from build123d import *

# Parameters (mm, degrees)
SKETCH_W                   = 21.1
SKETCH_H                   = 43.6
PAD_DEPTH                  = 3
SKETCH004_W                = 23.1
SKETCH004_H                = 45.6
PAD001_DEPTH               = 3
SKETCH005_W                = 7.05
SKETCH005_H                = 1.1
PAD002_DEPTH               = 5
SKETCH005_MIRRORED002_2_W  = 7.05
SKETCH005_MIRRORED002_2_H  = 1.1
PAD002_MIRRORED002_2_DEPTH = 5
SKETCH002_W                = 4.6
SKETCH002_H                = 9.5
POCKET_DEPTH               = 1
SKETCH001_R                = 1.65
POCKET001_DEPTH            = 0.001
POCKET001_DEPTH_BACK       = -5.001
SKETCH003_W                = 4
SKETCH003_H                = 4
POCKET002_DEPTH            = 2
SKETCH003_MIRRORED_2_W     = 4
SKETCH003_MIRRORED_2_H     = 4
POCKET002_MIRRORED_2_DEPTH = 2


with BuildPart() as part:
    # Sketch → Pad (new body)
    with BuildSketch(Plane.XY):
        Rectangle(SKETCH_W, SKETCH_H)
    extrude(amount=PAD_DEPTH)

    # Sketch004 → Pad001 (join)
    with BuildSketch(Plane.XY):
        Rectangle(SKETCH004_W, SKETCH004_H)
    extrude(amount=PAD001_DEPTH)

    # Sketch005 → Pad002 (join)
    with BuildSketch(Plane.XY):
        with Locations((3.525, 23.35)):
            Rectangle(SKETCH005_W, SKETCH005_H)
        Polygon((11.55, 22.8), (10.55, 22.8), (10.55, 23.9), (12.65, 23.9), (12.65, 0), (11.55, 0), align=None)
    pad002 = extrude(amount=PAD002_DEPTH)

    # Sketch005 Mirrored002 2 → Pad002 Mirrored002 2 (add)
    with BuildSketch(Plane(origin=(0, 0, 0), x_dir=(-1, 0, 0), z_dir=(0, 0, -1))):
        with Locations((3.525, 23.35)):
            Rectangle(SKETCH005_MIRRORED002_2_W, SKETCH005_MIRRORED002_2_H)
        Polygon((11.55, 22.8), (10.55, 22.8), (10.55, 23.9), (12.65, 23.9), (12.65, 0), (11.55, 0), align=None)
    pad002_mirrored002_2 = extrude(amount=-PAD002_MIRRORED002_2_DEPTH)

    # Mirrored003: Pad002, Pad002 Mirrored002 2 across Sketch005 H_Axis
    add(pad002.mirror(Plane.ZX))
    add(pad002_mirrored002_2.mirror(Plane.ZX))

    # Sketch002 → Pocket (cut)
    with BuildSketch(Plane(origin=(-8.2, 8.2, 3), x_dir=(1, 0, 0), z_dir=(0, 0, 1))):
        Rectangle(SKETCH002_W, SKETCH002_H)
    extrude(amount=-POCKET_DEPTH, mode=Mode.SUBTRACT)

    # Sketch001 → Pocket001 (cut, two sides)
    with BuildSketch(Plane.XY) as pocket001_sk:
        with Locations((7.643116, 15)):
            Circle(SKETCH001_R)
        with Locations((-7.643116, -15)):
            Circle(SKETCH001_R)
    extrude(amount=-POCKET001_DEPTH, mode=Mode.SUBTRACT)
    extrude(pocket001_sk.sketch, amount=-POCKET001_DEPTH_BACK, mode=Mode.SUBTRACT)

    # Sketch003 → Pocket002 (cut)
    with BuildSketch(Plane.XY.offset(3)):
        with Locations((8.55, 19.8)):
            Rectangle(SKETCH003_W, SKETCH003_H)
    pocket002 = extrude(amount=-POCKET002_DEPTH, mode=Mode.SUBTRACT)

    # Sketch003 Mirrored 2 → Pocket002 Mirrored 2 (cut)
    with BuildSketch(Plane(origin=(0, 0, 3), x_dir=(-1, 0, 0), z_dir=(0, 0, -1))):
        with Locations((8.55, 19.8)):
            Rectangle(SKETCH003_MIRRORED_2_W, SKETCH003_MIRRORED_2_H)
    pocket002_mirrored_2 = extrude(amount=POCKET002_MIRRORED_2_DEPTH, mode=Mode.SUBTRACT)

    # Mirrored001: Pocket002, Pocket002 Mirrored 2 across Sketch003 H_Axis
    add(pocket002.mirror(Plane(origin=(0, 0, 3), x_dir=(0, 0, 1), z_dir=(0, 1, 0))), mode=Mode.SUBTRACT)
    add(pocket002_mirrored_2.mirror(Plane(origin=(0, 0, 3), x_dir=(0, 0, 1), z_dir=(0, 1, 0))), mode=Mode.SUBTRACT)


solid = part.part
Geometry: final body of the model. Coordinates: model frame, mm. A direction names the side the tool comes from. Coordinates: 2 decimals unless noted, no trailing zeros. Order: outer loops, then holes, each group sorted by start corner. A loop starts at its lowest first (then second) coordinate and runs counter-clockwise, first axis right, second up. Notation, with made-up numbers: M 60.5,-0.5 L 93.5,-0.5 A22 cw 93.5,27.5 Z; hole C -40,12.5 d11. An arc over 180 degrees is marked long. One line per question, with ' | ' between items. Start each with the question number.
Item 1: Cut plane B-B, the plane x = 3. Return the cut outline in (y, z), then the cut area to 3 significant figures.
Item 2: Cut plane D-D, the plane y = 6. Return the cut outline in (x, z).
Item 3: Cut plane A-A, the plane z = 4.05. Return the cut outline in (x, y), then the cut area to 3 significant figures.
Item 4: Ray query, probe 1 along Y at (x, z) = (10.5, 1.3); probe 2 along X at (y, z) = (-8, 4.85); probe 3 along X at (y, z) = (-15, 1.35). Return the intervals inside material, ascending. Write a range as [from, to].
Item 5: Set-up query: faces 5 (the flat face through (7.05, -23, 2)), 6 (the flat face through (7.05, 23, 2)), 7 (the flat face through (-8, 8, 2)). Return all of +Z, -Z, +X, -X, +Y, -Y with unobstructed straight access to the full face (end or side cutting, diameter ignored); none if empty.
Item 6: Cut plane C-C, the plane y = -15. Return the cut outline in (x, z).
Item 7: Pin query (flat end, axial travel): pin 1 Ø1.1 at (x, z) = (-8.5, 2.5) entering from +Y; pin 2 Ø10 at (x, y) = (-3, -9.5) entering from +Z; pin 3 Ø2 at (x, y) = (9, -20) entering from +Z; pin 4 Ø5.5 at (x, y) = (-7.64, -15) entering from -Z. Return the tip coordinate at first contact, or that it passes through.
Item 8: Draft query along Y for faces 1 (the flat face through (11, -22.8, 4)), 2 (the flat face through (6.55, 20, 2)), 3 (the flat face through (-9, 22.8, 1)), 4 (the flat face through (0, 0, 0)). Return one class per face: released by +Y, released by -Y, zero draft, split by the parting line, or undercut.
A:
1) outline: M -23.9,0 L 23.9,0 L 23.9,5 L 22.8,5 L 22.8,3 L -22.8,3 L -22.8,5 L -23.9,5 Z | area: 148 mm2
2) outline: M -12.65,0 L 12.65,0 L 12.65,5 L 11.55,5 L 11.55,3 L -5.9,3 L -5.9,2 L -10.5,2 L -10.5,3 L -11.55,3 L -11.55,5 L -12.65,5 Z
3) outline: M -12.65,-23.9 L -10.55,-23.9 L -10.55,-22.8 L -11.55,-22.8 L -11.55,22.8 L -10.55,22.8 L -10.55,23.9 L -12.65,23.9 Z; M -7.05,-23.9 L 7.05,-23.9 L 7.05,-22.8 L -7.05,-22.8 Z; M -7.05,22.8 L 7.05,22.8 L 7.05,23.9 L -7.05,23.9 Z; M 10.55,-23.9 L 12.65,-23.9 L 12.65,23.9 L 10.55,23.9 L 10.55,22.8 L 11.55,22.8 L 11.55,-22.8 L 10.55,-22.8 Z | area: 141 mm2
4) probe 1: y = [-22.8, -21.8], [-17.8, 17.8], [21.8, 22.8] | probe 2: x = [-12.65, -11.55], [11.55, 12.65] | probe 3: x = [-12.65, -9.29], [-5.99, 12.65]
5) face 5: +Z, -Z, -Y | face 6: +Z, -Z, +Y | face 7: +Z
6) outline: M -12.65,0 L -9.29,0 L -9.29,3 L -11.55,3 L -11.55,5 L -12.65,5 Z; M -5.99,0 L 12.65,0 L 12.65,5 L 11.55,5 L 11.55,3 L -5.99,3 Z
7) pin 1: stops at y = 22.8 | pin 2: stops at z = 3 | pin 3: stops at z = 1 | pin 4: stops at z = 0
8) face 1: undercut | face 2: undercut | face 3: released by +Y | face 4: zero draft
